from build123d import *

# Parameters (mm, degrees)
F0_R     = 12.5
F1_DEPTH = 200
F2_R     = 5
F3_DEPTH = 10
F4_R     = 5
F5_DEPTH = 10
F6_R     = 5
F7_R     = 5


with BuildPart() as f1:
    # F0 (on Front) → F1 (new body)
    with BuildSketch(Plane.XZ):
        Circle(F0_R)
    extrude(amount=F1_DEPTH)

    # F2 (on face) → F3 (join)
    with BuildSketch(Plane.XZ.offset(200)):
        Circle(F2_R)
    extrude(amount=F3_DEPTH)

    # F4 (on face) → F5 (join)
    with BuildSketch(Plane(origin=(0, 0, 0), x_dir=(-1, 0, 0), z_dir=(0, 1, 0))):
        Circle(F4_R)
    extrude(amount=F5_DEPTH)

    # F6
    f6_edges = [f1.edges().sort_by_distance(p)[0] for p in [
        (-12.5, -200, 0),
    ]]
    fillet(f6_edges, radius=F6_R)

    # F7
    f7_edges = [f1.edges().sort_by_distance(p)[0] for p in [
        (-12.5, 0, 0),
        (11.035534, -198.535534, 0),
        (-12.5, -195, 0),
        (-7.5, -200, 0),
    ]]
    fillet(f7_edges, radius=F7_R)


solid = f1.part
Could you check a few things on this model? Use its own coordinates, in mm. A direction names the side the tool comes from. Give positions to 0.01 mm unless a question says otherwise; leave off trailing zeros. Order: outer loops, then holes, each group sorted by start corner. A loop starts at its lowest first (then second) coordinate and runs counter-clockwise, first axis right, second up.
Item 1: For faces 1 (the face through (1.08, 4.93, -4.88)), 2 (the face through (-1.08, -204.93, -4.88)), 3 (the face through (0, 10, 0)), which set-ups out of +Z, -Z, +X, -X, +Y, -Y let a thin tool reach every point of the face, with its end or its side?
Item 2: If we section it at C-C, the plane y = -114.5: Write out the boundary of the cut face in (x, z), plus the area to 3 significant figures.
Item 3: If we section it at B-B, the plane z = 0: Write out the boundary of the cut face in (x, y), plus the area to 3 significant figures.
Item 4: I'm going to push flat-ended pins straight in: pin 1 (1 mm diameter, centred on y = -56, z = 2.5, fed in from -X); pin 2 (8 mm diameter, centred on y = -61, z = -7, fed in from +X); pin 3 (10 mm diameter, centred on x = 7.5, y = -142.5, fed in from -Z). Where does each tip first touch, or does it pass through?
Item 5: If we section it at A-A, the plane x = 0: Write out the boundary of the cut face in (y, z).
Item 6: I need wall thicknesses on line 1 (Z direction, x = 10, y = -71); line 2 (Y direction, x = -4.5, z = -4.5); line 3 (Z direction, x = -0.5, y = -51). Which ranges of each line are inside material? Lowest first, please.
Values:
1. face 1: +Y
1. face 2: -Y
1. face 3: +Z, -Z, +X, -X, +Y
2. outline: circle Ø25 at (0, 0)
2. area: 491 mm2
3. outline: (-12.5, -195) arc R5 ccw to (-7.5, -200) - (-5, -200) - (-5, -210) - (5, -210) - (5, -200) - (7.5, -200) arc R5 ccw to (12.5, -195) - (12.5, -5) arc R5 ccw to (7.5, 0) - (5, 0) - (5, 10) - (-5, 10) - (-5, 0) - (-7.5, 0) arc R5 ccw to (-12.5, -5) - close
3. area: 5,180 mm2
4. pin 1: stops at x = -12.34
4. pin 2: stops at x = 12.13
4. pin 3: stops at z = -12.25
5. outline: (-210, -5) - (-200, -5) - (-200, -7.5) arc R5 ccw to (-195, -12.5) - (-5, -12.5) arc R5 ccw to (0, -7.5) - (0, -5) - (10, -5) - (10, 5) - (0, 5) - (0, 7.5) arc R5 ccw to (-5, 12.5) - (-195, 12.5) arc R5 ccw to (-200, 7.5) - (-200, 5) - (-210, 5) - close
6. line 1: z = -7.5 to 7.5
6. line 2: y = -200 to 0
6. line 3: z = -12.49 to 12.49
